Geometry check sheet. Reference: the model listing, model coordinates, mm. A direction names the side the tool comes from. Coordinates: 2 decimals unless noted, no trailing zeros. Loops run counter-clockwise (first coordinate to the right, second up) from the corner with the lowest first, then second, coordinate; pieces in that order, holes last. Notation, with made-up numbers: (83, 80) -> (100, 80) arc R28 cw to (100, 104) -> close; hole circle Ø11 at (-21, 61). An arc over 180 degrees is marked (long way). Answer as a JSON object with one key per item and string values.
from build123d import *

# Parameters (mm, degrees)
BOSS_EXTRUDE1_DEPTH      = 2.5
BOSS_EXTRUDE2_DEPTH      = 12.7
BOSS_EXTRUDE3_START      = 12.7
SKETCH3_W                = 11.9
SKETCH3_H                = 4.75
SKETCH3_W_2              = 10.75
BOSS_EXTRUDE3_DEPTH      = 12.7
BOSS_EXTRUDE4_START      = 25.4
SKETCH3_3_W              = 11.9
SKETCH3_3_H              = 4.75
SKETCH3_3_W_2            = 10.75
SKETCH3_3_W_3            = 1.15
BOSS_EXTRUDE4_DEPTH      = 2
CUT_EXTRUDE1_START       = -1.1
SKETCH2_R                = 1.05
CUT_EXTRUDE1_DEPTH       = 8
CUT_EXTRUDE2_START       = 3.1
SKETCH2_3_R              = 1.05
CUT_EXTRUDE2_DEPTH       = 8
BOSS_EXTRUDE5_START      = 7
SKETCH1_4_R              = 2.075
BOSS_EXTRUDE5_DEPTH      = 10
BOSS_EXTRUDE6_START      = 12.7
SKETCH1_7_W              = 7.7
SKETCH1_7_H              = 6.8
SKETCH1_7_R              = 2.075
BOSS_EXTRUDE6_DEPTH      = 10
FILLET1_R                = 2
CUT_EXTRUDE3_START       = 12.7
SKETCH5_W                = 14.55
SKETCH5_H                = 4.75
CUT_EXTRUDE3_DEPTH       = 2
CUT_EXTRUDE4_START       = 12.7
SKETCH6_W                = 7.7
SKETCH6_H                = 4.75
CUT_EXTRUDE4_DEPTH       = 4
BOSS_EXTRUDE7_DEPTH      = 2.5
BOSS_EXTRUDE7_DEPTH_BACK = 2
BOSS_EXTRUDE7_START      = 27.4
SKETCH7_W                = 4
SKETCH7_H                = 15
SKETCH7_W_2              = 5
SKETCH7_H_2              = 5
SKETCH7_R                = 1.05
SKETCH7_W_3              = 2.5


with BuildPart() as part:
    # Sketch1 → Boss-Extrude1 (new body)
    with BuildSketch(Plane(origin=(0, 0, 0), x_dir=(1, 0, 0), z_dir=(0, 1, 0))):
        Polygon((-1.1, 16.25), (-1.1, -16.25), (8.9, -16.25), (8.9, -11.5), (17.65, -11.5), (17.65, 16.25), align=None)
    extrude(amount=-BOSS_EXTRUDE1_DEPTH)

    # Sketch1<3> → Boss-Extrude2 (add)
    with BuildSketch(Plane(origin=(0, 0, 0), x_dir=(1, 0, 0), z_dir=(0, 1, 0))):
        Polygon((9.9, 16.25), (-1.1, 16.25), (-1.1, 11.5), (17.65, 11.5), (17.65, 16.25), (17.6, 16.25), align=None)
        Polygon((8.9, -11.5), (-1.1, -11.5), (-1.1, -16.25), (2.35, -16.25), (8.9, -16.25), align=None)
    extrude(amount=BOSS_EXTRUDE2_DEPTH)

    # Sketch3 → Boss-Extrude3 (add)
    with BuildSketch(Plane(origin=(0, 0, 0), x_dir=(1, 0, 0), z_dir=(0, 1, 0)).offset(BOSS_EXTRUDE3_START)):
        with Locations((-2.85, 13.875)):
            Rectangle(SKETCH3_W, SKETCH3_H)
        with Locations((-2.275, -13.875)):
            Rectangle(SKETCH3_W_2, SKETCH3_H)
    extrude(amount=BOSS_EXTRUDE3_DEPTH)

    # Sketch3<3> → Boss-Extrude4 (add)
    with BuildSketch(Plane(origin=(0, 0, 0), x_dir=(1, 0, 0), z_dir=(0, 1, 0)).offset(BOSS_EXTRUDE4_START)):
        with Locations((-2.85, 13.875)):
            Rectangle(SKETCH3_3_W, SKETCH3_3_H)
        Polygon((3.1, -11.5), (3.1, 11.5), (-8.8, 11.5), (-8.8, -11.5), (-7.65, -11.5), align=None)
        with Locations((-2.275, -13.875)):
            Rectangle(SKETCH3_3_W_2, SKETCH3_3_H)
        with Locations((-8.225, -13.875)):
            Rectangle(SKETCH3_3_W_3, SKETCH3_3_H)
    extrude(amount=BOSS_EXTRUDE4_DEPTH)

    # Sketch2 → Cut-Extrude1 (cut)
    with BuildSketch(Plane(origin=(0, 0, 0), x_dir=(0, 0, -1), z_dir=(1, 0, 0)).offset(CUT_EXTRUDE1_START)):
        with Locations(Location((-13.7, 6.45, 0), (0, 0, 180))):
            Circle(SKETCH2_R)
        with Locations(Location((13.7, 6.45, 0), (0, 0, 180))):
            Circle(SKETCH2_R)
    extrude(amount=CUT_EXTRUDE1_DEPTH, mode=Mode.SUBTRACT)

    # Sketch2<3> → Cut-Extrude2 (cut)
    with BuildSketch(Plane(origin=(0, 0, 0), x_dir=(0, 0, -1), z_dir=(1, 0, 0)).offset(CUT_EXTRUDE2_START)):
        with Locations(Location((13.7, 19.15, 0), (0, 0, 180))):
            Circle(SKETCH2_3_R)
        with Locations(Location((-13.7, 19.15, 0), (0, 0, 180))):
            Circle(SKETCH2_3_R)
    extrude(amount=-CUT_EXTRUDE2_DEPTH, mode=Mode.SUBTRACT)

    # Sketch1<4> → Boss-Extrude5 (add)
    with BuildSketch(Plane(origin=(0, 0, 0), x_dir=(1, 0, 0), z_dir=(0, 1, 0)).offset(BOSS_EXTRUDE5_START)):
        Polygon((2.35, -16.25), (-1.1, -16.25), (-3.8, -16.25), (-5.35, -16.25), (-5.35, -23.05), (2.35, -23.05), align=None)
        with Locations(Location((-1.5, -19.85, 0), (0, 0, 270))):
            Circle(SKETCH1_4_R, mode=Mode.SUBTRACT)
    extrude(amount=BOSS_EXTRUDE5_DEPTH)

    # Sketch1<7> → Boss-Extrude6 (add)
    with BuildSketch(Plane(origin=(0, 0, 0), x_dir=(1, 0, 0), z_dir=(0, 1, 0)).offset(BOSS_EXTRUDE6_START)):
        with Locations((13.75, 19.65)):
            Rectangle(SKETCH1_7_W, SKETCH1_7_H)
        with Locations(Location((13.75, 19.85, 0), (0, 0, 270))):
            Circle(SKETCH1_7_R, mode=Mode.SUBTRACT)
    extrude(amount=-BOSS_EXTRUDE6_DEPTH)

    # Fillet1
    fillet1_edges = [part.edges().sort_by_distance(p)[0] for p in [
        (3.9, -2.5, 16.25),
        (-2.85, 27.4, 16.25),
        (8.275, -2.5, -16.25),
        (-2.85, 27.4, -16.25),
    ]]
    fillet(fillet1_edges, radius=FILLET1_R)

    # Sketch5 → Cut-Extrude3 (cut)
    with BuildSketch(Plane(origin=(0, 0, 0), x_dir=(1, 0, 0), z_dir=(0, 1, 0)).offset(CUT_EXTRUDE3_START)):
        with Locations((10.375, 13.875)):
            Rectangle(SKETCH5_W, SKETCH5_H)
    extrude(amount=-CUT_EXTRUDE3_DEPTH, mode=Mode.SUBTRACT)

    # Sketch6 → Cut-Extrude4 (cut)
    with BuildSketch(Plane(origin=(0, 0, 0), x_dir=(1, 0, 0), z_dir=(0, 1, 0)).offset(CUT_EXTRUDE4_START)):
        with Locations((-4.95, 13.875)):
            Rectangle(SKETCH6_W, SKETCH6_H)
    extrude(amount=CUT_EXTRUDE4_DEPTH, mode=Mode.SUBTRACT)

    # Sketch7 → Boss-Extrude7 (add, two sides: drawn at the far end of the back side and taken through both)
    # profile 1 of 5: a face of its own
    with BuildSketch(Plane(origin=(0, 0, 0), x_dir=(1, 0, 0), z_dir=(0, 1, 0)).offset(BOSS_EXTRUDE7_START - BOSS_EXTRUDE7_DEPTH_BACK)):
        with Locations((-3, 0)):
            Rectangle(SKETCH7_W, SKETCH7_H)
    # profile 2 of 5: a face of its own
    with BuildSketch(Plane(origin=(0, 0, 0), x_dir=(1, 0, 0), z_dir=(0, 1, 0)).offset(BOSS_EXTRUDE7_START - BOSS_EXTRUDE7_DEPTH_BACK)):
        with Locations((4, -11.43)):
            Rectangle(SKETCH7_W_2, SKETCH7_H_2)
        with Locations(Location((4, -11.43, 0), (0, 0, 211.002719134))):
            Circle(SKETCH7_R, mode=Mode.SUBTRACT)
    # profile 3 of 5: a face of its own
    with BuildSketch(Plane(origin=(0, 0, 0), x_dir=(1, 0, 0), z_dir=(0, 1, 0)).offset(BOSS_EXTRUDE7_START - BOSS_EXTRUDE7_DEPTH_BACK)):
        with Locations((0.25, -11.43)):
            Rectangle(SKETCH7_W_3, SKETCH7_H_2)
    # profile 4 of 5: a face of its own
    with BuildSketch(Plane(origin=(0, 0, 0), x_dir=(1, 0, 0), z_dir=(0, 1, 0)).offset(BOSS_EXTRUDE7_START - BOSS_EXTRUDE7_DEPTH_BACK)):
        with Locations((0.25, 11.43)):
            Rectangle(SKETCH7_W_3, SKETCH7_H_2)
    # profile 5 of 5: a face of its own
    with BuildSketch(Plane(origin=(0, 0, 0), x_dir=(1, 0, 0), z_dir=(0, 1, 0)).offset(BOSS_EXTRUDE7_START - BOSS_EXTRUDE7_DEPTH_BACK)):
        with Locations((4, 11.43)):
            Rectangle(SKETCH7_W_2, SKETCH7_H_2)
        with Locations(Location((4, 11.43, 0), (0, 0, 211.002719134))):
            Circle(SKETCH7_R, mode=Mode.SUBTRACT)
    extrude(amount=BOSS_EXTRUDE7_DEPTH + BOSS_EXTRUDE7_DEPTH_BACK)


solid = part.part
1. Mould release check, pull along Y, two halves, no side actions. Record for faces 4 (the face through (-4.9, 19, 14)), 5 (the face through (6.5, 28, -11)), 6 (the face through (2.7, 29.9, -11.5)): released by +Y, released by -Y, zero draft, split by the parting line, or undercut.
Evaluation:
{"face 4": "undercut", "face 5": "zero draft", "face 6": "released by +Y"}
2. Depth check by flat-ended pin: P1, Ø1.4, axis at y = 17, z = 14, coming from the -X side; P2, Ø4.5, axis at y = 18.5, z = 14.5, coming from the +X side; P3, Ø5.5, axis at y = 12.5, z = 21, coming from the -X side. Enter the tip coordinate at first touch or a pass-through.
Evaluation:
{"P1": "stops at x = -7.65", "P2": "stops at x = 3.1", "P3": "stops at x = -5.35"}
3. Tool access check on faces 1 (the face through (1, 13, 11.5)), 2 (the face through (-0.84, 19.55, -12.73)), 3 (the face through (-5.35, 12, 20)). Record the directions out of +Z, -Z, +X, -X, +Y, -Y that give a thin tool (end or side, any length) a straight path to the whole face; none if there is none.
Evaluation:
{"face 1": "+X, -X", "face 2": "+X", "face 3": "+Z, -X, +Y, -Y"}
4. Section check C-C, the plane z = -9.5. Record the boundary of the cut face in (x, y), then the cut area to 3 significant figures.
Evaluation:
{"outline": "(-8.8, 25.4) -> (6.5, 25.4) -> (6.5, 29.9) -> (-1, 29.9) -> (-1, 27.4) -> (-8.8, 27.4) -> close; (-1.1, -2.5) -> (17.65, -2.5) -> (17.65, 0) -> (-1.1, 0) -> close", "area": "96.2 mm^2"}
5. Section check A-A, the plane y = 16. Record the boundary of the cut face in (x, z) (3 decimals).
Evaluation:
{"outline": "(-7.65, 11.5) -> (3.1, 11.5) -> (3.1, 16.25) -> (2.35, 16.25) -> (2.35, 23.05) -> (-5.35, 23.05) -> (-5.35, 16.25) -> (-7.65, 16.25) -> close; (-1.1, -16.25) -> (3.1, -16.25) -> (3.1, -11.5) -> (-1.1, -11.5) -> close; hole circle Ø4.15 at (-1.5, 19.85)"}
6. Section check B-B, the plane x = 4. Record the boundary of the cut face in (y, z).
Evaluation:
{"outline": "(-2.5, -14.25) arc R2 ccw to (-0.5, -16.25) -> (10.7, -16.25) -> (10.7, -11.5) -> (0, -11.5) -> (0, 11.5) -> (12.7, 11.5) -> (12.7, 16.25) -> (-0.5, 16.25) arc R2 ccw to (-2.5, 14.25) -> close; (25.4, -13.93) -> (29.9, -13.93) -> (29.9, -12.48) -> (25.4, -12.48) -> close; (25.4, -10.38) -> (29.9, -10.38) -> (29.9, -8.93) -> (25.4, -8.93) -> close; (25.4, 8.93) -> (29.9, 8.93) -> (29.9, 10.38) -> (25.4, 10.38) -> close; (25.4, 12.48) -> (29.9, 12.48) -> (29.9, 13.93) -> (25.4, 13.93) -> close; hole circle Ø2.1 at (6.45, -13.7); hole circle Ø2.1 at (6.45, 13.7)"}
7. Section check D-D, the plane y = 11.5. Record the boundary of the cut face in (x, z) (3 decimals).
Evaluation:
{"outline": "(-5.35, 16.25) -> (-1.1, 16.25) -> (-1.1, 11.5) -> (8.9, 11.5) -> (8.9, 16.25) -> (2.35, 16.25) -> (2.35, 23.05) -> (-5.35, 23.05) -> close; (-1.1, -16.25) -> (3.1, -16.25) -> (3.1, -11.5) -> (-1.1, -11.5) -> close; (9.9, -23.05) -> (17.6, -23.05) -> (17.6, -16.25) -> (9.9, -16.25) -> close; hole circle Ø4.15 at (-1.5, 19.85); hole circle Ø4.15 at (13.75, -19.85)"}
8. Thickness scan on probe 1 along Z at (x, y) = (2.5, 6.45); probe 2 along Y at (x, z) = (0.75, -13.7); probe 3 along Y at (x, z) = (4.5, 13.7). Record the ranges inside material, lowest first. Write a range as from..to.
Evaluation:
{"probe 1": "z = -16.25..-14.75, -12.65..-11.5, 11.5..12.65, 14.75..16.25", "probe 2": "y = -2.5..5.4, 7.5..18.1, 20.2..29.9", "probe 3": "y = -2.5..5.4, 7.5..12.7, 25.4..29.9"}
